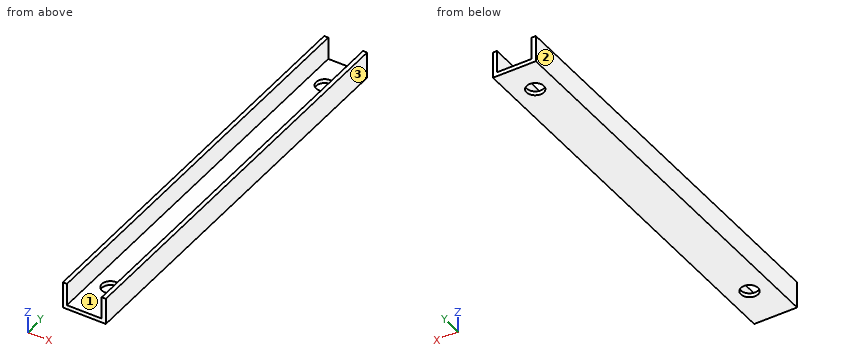
```python
from build123d import *

# Parameters (mm, degrees)
EXTRUDE_THIN1_DEPTH = 100
SKETCH2_R           = 2.1
CUT_EXTRUDE1_DEPTH  = 10


with BuildPart() as part:
    # Sketch1 → Extrude-Thin1 (new body)
    with BuildSketch(Plane(origin=(0, 0, 0), x_dir=(1, 0, 0), z_dir=(0, 1, 0))):
        Polygon((-3.469957082, -1.813304721), (-3.469957082, 4.686695279), (7.030042918, 4.686695279), (7.030042918, -1.813304721), (6.030042918, -1.813304721), (6.030042918, 3.686695279), (-2.469957082, 3.686695279), (-2.469957082, -1.813304721), align=None)
    extrude(amount=EXTRUDE_THIN1_DEPTH)

    # Sketch2 → Cut-Extrude1 (cut)
    with BuildSketch(Plane(origin=(0, 0, -4.686695279), x_dir=(-1, 0, 0), z_dir=(0, 0, -1))):
        with Locations((-1.780042918, 92)):
            Circle(SKETCH2_R)
        with Locations((-1.780042918, 10)):
            Circle(SKETCH2_R)
    extrude(amount=-CUT_EXTRUDE1_DEPTH, mode=Mode.SUBTRACT)


solid = part.part
```
Work out the finished part from the listing and answer in its coordinate system (mm). Face numbers are marked on the shaded views. Coordinates: 2 decimals unless noted, no trailing zeros. Write each loop counter-clockwise with the first axis right and the second up, starting at its lowest first coordinate (ties: lowest second). Pieces come first, ordered by that corner, then holes.
Q1. A cutting plane is placed at A-A, the plane z = -2.25. Give the vertices of the cut face in (x, y).
Q2. Determine the mould class of the marked faces 1, 2 and 3 for opening direction X: released by +X, released by -X, zero draft, split by the parting line, or undercut.
Q3. Find the intervals of material crossed by line 1 (X direction, y = 61, z = -1); line 2 (Z direction, x = 4, y = 31.5), in increasing order.
Q4. Each of these flat-tipped pins is pushed along its axis until it touches: pin 1 Ø3 at (x, z) = (-2, 0) entering from +Y; pin 2 Ø4 at (x, y) = (0, 60.5) entering from +Z. Where does it stop, or does it pass through?
Q5. A cutting plane is placed at B-B, the plane y = 10. Give the vertices of the cut face in (x, z), then the cut area to 3 significant figures.
Q6. A cutting plane is placed at C-C, the plane y = 78. Give the vertices of the cut face in (x, z).
Q7. A cutting plane is placed at D-D, the plane x = 5. Give the vertices of the cut face in (y, z).
Findings below:
1. outline: (-3.47, 0) - (-2.47, 0) - (-2.47, 100) - (-3.47, 100) - close; (6.03, 0) - (7.03, 0) - (7.03, 100) - (6.03, 100) - close
2. face 1: undercut
2. face 2: released by -X
2. face 3: released by +X
3. line 1: x = -3.47 to -2.47, 6.03 to 7.03
3. line 2: z = -4.69 to -3.69
4. pin 1: stops at y = 100
4. pin 2: stops at z = -3.69
5. outline: (-3.47, -4.69) - (-0.32, -4.69) - (-0.32, -3.69) - (-2.47, -3.69) - (-2.47, 1.81) - (-3.47, 1.81) - close; (3.88, -4.69) - (7.03, -4.69) - (7.03, 1.81) - (6.03, 1.81) - (6.03, -3.69) - (3.88, -3.69) - close
5. area: 17.3 mm2
6. outline: (-3.47, -4.69) - (7.03, -4.69) - (7.03, 1.81) - (6.03, 1.81) - (6.03, -3.69) - (-2.47, -3.69) - (-2.47, 1.81) - (-3.47, 1.81) - close
7. outline: (0, -4.69) - (100, -4.69) - (100, -3.69) - (0, -3.69) - close
